Source: CAD feature listing. Evaluate the final solid. Frame: model axes, mm. A direction names the side the tool comes from. Give positions to 0.01 mm unless a question says otherwise; leave off trailing zeros. Loops run counter-clockwise (first coordinate to the right, second up) from the corner with the lowest first, then second, coordinate; pieces in that order, holes last. Notation, with made-up numbers: M -31.75,-29 L 13.25,-29 A17 cw 13.25,-9 Z; hole C -27,42.5 d2. An arc over 180 degrees is marked long. Write item = value, one per line.
from build123d import *

# Parameters (mm, degrees)
F0_R     = 8.89
F1_DEPTH = 25.4
F2_DEPTH = 44.45


with BuildPart() as f1:
    # F0 (on Front) → F1 (new body)
    with BuildSketch(Plane.XZ):
        with BuildLine():
            ThreePointArc((-6.6145833333, -31.0533377808), (19.97560361, -24.6786904113), (31.75, 0))
            ThreePointArc((31.75, 0), (19.97560361, 24.6786904113), (-6.6145833333, 31.0533377808))
            ThreePointArc((-6.6145833333, 31.0533377808), (-31.75, 0), (-6.6145833333, -31.0533377808))
        make_face()
        with BuildLine():
            ThreePointArc((-8.1752396754, 3.4925), (0, 8.89), (8.1752396754, 3.4925))
            Line((8.1752396754, 3.4925), (15.875, 3.4925))
            Line((15.875, 3.4925), (15.875, -3.4925))
            Line((15.875, -3.4925), (8.1752396754, -3.4925))
            ThreePointArc((8.1752396754, -3.4925), (0, -8.89), (-8.1752396754, -3.4925))
            Line((-8.1752396754, -3.4925), (-15.875, -3.4925))
            Line((-15.875, -3.4925), (-15.875, 3.4925))
            Line((-15.875, 3.4925), (-8.1752396754, 3.4925))
        make_face(mode=Mode.SUBTRACT)
        with BuildLine():
            ThreePointArc((-6.6145833333, -31.0533377808), (-31.75, 0), (-6.6145833333, 31.0533377808))
            Line((-6.6145833333, 31.0533377808), (-79.5072916667, 15.5266688904))
            ThreePointArc((-79.5072916667, 15.5266688904), (-66.212198195, 12.3393452056), (-60.325, 0))
            ThreePointArc((-60.325, 0), (-66.212198195, -12.3393452056), (-79.5072916667, -15.5266688904))
            Line((-79.5072916667, -15.5266688904), (-6.6145833333, -31.0533377808))
        make_face()
        with BuildLine():
            ThreePointArc((-60.325, 0), (-66.212198195, 12.3393452056), (-79.5072916667, 15.5266688904))
            ThreePointArc((-79.5072916667, 15.5266688904), (-92.075, 0), (-79.5072916667, -15.5266688904))
            ThreePointArc((-79.5072916667, -15.5266688904), (-66.212198195, -12.3393452056), (-60.325, 0))
        make_face()
        with Locations((-76.2, 0)):
            Circle(F0_R, mode=Mode.SUBTRACT)
        with BuildLine():
            ThreePointArc((-8.1752396754, -3.4925), (-8.89, 0), (-8.1752396754, 3.4925))
            Line((-8.1752396754, 3.4925), (-15.875, 3.4925))
            Line((-15.875, 3.4925), (-15.875, -3.4925))
            Line((-15.875, -3.4925), (-8.1752396754, -3.4925))
        make_face()
    extrude(amount=F1_DEPTH)

    # F0 (on Front) → F2 (join)
    with BuildSketch(Plane.XZ):
        with BuildLine():
            ThreePointArc((-6.6145833333, -31.0533377808), (19.97560361, -24.6786904113), (31.75, 0))
            ThreePointArc((31.75, 0), (19.97560361, 24.6786904113), (-6.6145833333, 31.0533377808))
            ThreePointArc((-6.6145833333, 31.0533377808), (-31.75, 0), (-6.6145833333, -31.0533377808))
        make_face()
        with BuildLine():
            ThreePointArc((-8.1752396754, 3.4925), (0, 8.89), (8.1752396754, 3.4925))
            Line((8.1752396754, 3.4925), (15.875, 3.4925))
            Line((15.875, 3.4925), (15.875, -3.4925))
            Line((15.875, -3.4925), (8.1752396754, -3.4925))
            ThreePointArc((8.1752396754, -3.4925), (0, -8.89), (-8.1752396754, -3.4925))
            Line((-8.1752396754, -3.4925), (-15.875, -3.4925))
            Line((-15.875, -3.4925), (-15.875, 3.4925))
            Line((-15.875, 3.4925), (-8.1752396754, 3.4925))
        make_face(mode=Mode.SUBTRACT)
        with BuildLine():
            ThreePointArc((-8.1752396754, -3.4925), (-8.89, 0), (-8.1752396754, 3.4925))
            Line((-8.1752396754, 3.4925), (-15.875, 3.4925))
            Line((-15.875, 3.4925), (-15.875, -3.4925))
            Line((-15.875, -3.4925), (-8.1752396754, -3.4925))
        make_face()
    extrude(amount=F2_DEPTH)


solid = f1.part
1. Cut plane B-B, the plane z = 0. Return the cut outline in (x, y) (3 decimals).
Derived:
outline = M -92.075,-25.4 L -85.09,-25.4 L -85.09,0 L -92.075,0 Z; M -67.31,-25.4 L -31.75,-25.4 L -31.75,-44.45 L -8.89,-44.45 L -8.89,0 L -67.31,0 Z; M 15.875,-44.45 L 31.75,-44.45 L 31.75,0 L 15.875,0 Z
2. Cut plane A-A, the plane x = 0. Return the cut outline in (y, z).
Derived:
outline = M -44.45,-31.75 L 0,-31.75 L 0,-8.89 L -44.45,-8.89 Z; M -44.45,8.89 L 0,8.89 L 0,31.75 L -44.45,31.75 Z
3. First-contact query: pin 1 Ø10 at (y, z) = (-10.5, 9) entering from +X; pin 2 Ø7.5 at (y, z) = (-29.5, 1) entering from -X; pin 3 Ø5 at (y, z) = (-15, 13.5) entering from -X. Flat tips, straight axial feed; report the tip coordinate or a pass-through.
Derived:
pin_1 = 31.5
pin_2 = -31.75
pin_3 = -87.65
4. Material intervals for probe 1 along X at (y, z) = (-3, 5.5); probe 2 along Y at (x, z) = (-60.5, 1.5); probe 3 along Z at (x, y) = (-7.5, -33), sorted ascending. Write a range as from..to.
Derived:
probe_1 = -91.09..-83.18, -69.22..-6.98, 6.98..31.27
probe_2 = -25.4..0
probe_3 = -30.85..-4.77, 4.77..30.85
5. Reachability of faces 5 (the cylindrical face through (31.75, -26.85, -0.27)), 6 (the cylindrical face through (-92.072, -12.522, 0.302)), 7 (the flat face through (12, -22, 3.492)) from +Z, -Z, +X, -X, +Y, -Y: full face, straight path, thin tool, end or side. Return the list, or none.
Derived:
face_5 = -Y
face_6 = -X, +Y, -Y
face_7 = +Y, -Y
6. Cut plane C-C, the plane y = -10. Count the separate pieces of the cut face and the enclosed holes in it, then the cut area to 3 significant figures.
Derived:
separate_pieces = 1
enclosed_holes = 2
area = 5,140 mm²
7. Pull-direction query (X, two-part tool) for faces 1 (the flat face through (-50, -25.4, 0)), 2 (the cylindrical face through (-67.72, -12.52, 2.67)), 3 (the flat face through (-42.55, -12.52, 23.4)), 4 (the flat face through (15.875, -22, 0)); classes: +X half, -X half, draft (parallel to the pull), parting line (faces both ways), or undercut.
Derived:
face_1 = draft
face_2 = undercut
face_3 = -X half
face_4 = undercut
